The listing builds one solid part. Answer for the finished solid, in the listing's coordinates (mm). Coordinates: 2 decimals unless noted, no trailing zeros. Loops run counter-clockwise (first coordinate to the right, second up) from the corner with the lowest first, then second, coordinate; pieces in that order, holes last. Notation, with made-up numbers: M 31.5,-28 L 56.5,-28 A19 ccw 56.5,7 Z; hole C 42.25,13 d10. An arc over 180 degrees is marked long. Return JSON: item names as keys, results as strings. Group by question number.
1. Section A-A (y = -16) is taken. Write down the section's boundary in (x, z).
2. Section D-D (z = 4.1) is taken. Count the separate pieces of the cut face and the enclosed holes in it, then the cut area to 3 significant figures.
3. Given P1, Ø3.5, axis at x = 3.5, y = 1.5, coming from the +Z side, flat-ended and moving along its own axis, determine where the tip first touches the part or whether it passes through.
4. Straight lines are drawn through the part: L1, parallel to Y at x = 28, z = 3.2; L2, parallel to Y at x = 4, z = 2.1; L3, parallel to Y at x = -38.5, z = 4.05. For each, find the intervals that lie inside material, in ascending order. Write a range as from..to.
5. Section C-C (x = 15) is taken. Write down the section's boundary in (y, z).
6. Section B-B (x = -32) is taken. Write down the section's boundary in (y, z), then the cut area to 3 significant figures.
```python
from build123d import *

# Parameters (mm, degrees)
SKETCH_1_W          = 100
SKETCH_1_H          = 100
SKETCH_1_R          = 1.5
EXTRUDE_1_DEPTH     = 5
SKETCH_2_R          = 1
CUT_EXTRUDE_1_DEPTH = 71.887234394
SKETCH_3_R          = 3.5
CUT_EXTRUDE_2_DEPTH = 2
SKETCH_4_R          = 1.5
CUT_EXTRUDE_3_DEPTH = 10
SKETCH_5_R          = 1.5
CUT_EXTRUDE_4_DEPTH = 10
SKETCH_6_W          = 30
SKETCH_6_H          = 50
CUT_EXTRUDE_5_DEPTH = 10


with BuildPart() as part:
    # 草图1 → 凸台-拉伸1 (new body)
    with BuildSketch(Plane.XY):
        Rectangle(SKETCH_1_W, SKETCH_1_H)
        with Locations((-4, 0)):
            Circle(SKETCH_1_R, mode=Mode.SUBTRACT)
        with Locations(Location((4, 0, 0), (0, 0, 180))):
            Circle(SKETCH_1_R, mode=Mode.SUBTRACT)
    extrude(amount=EXTRUDE_1_DEPTH)

    # 草图2 → 切除-拉伸1 (cut, through all)
    with BuildSketch(Plane.XY.offset(5)):
        with Locations(Location((-46, -46, 0), (0, 0, 180))):
            Circle(SKETCH_2_R)
        with Locations((-46, 16)):
            Circle(SKETCH_2_R)
        with Locations((-4, -46)):
            Circle(SKETCH_2_R)
        with Locations((-4, 16)):
            Circle(SKETCH_2_R)
    extrude(amount=-CUT_EXTRUDE_1_DEPTH, mode=Mode.SUBTRACT)

    # 草图3 → 切除-拉伸2 (cut)
    with BuildSketch(Plane.XY.offset(5)):
        with Locations((-4, 0)):
            Circle(SKETCH_3_R)
        with Locations((4, 0)):
            Circle(SKETCH_3_R)
    extrude(amount=-CUT_EXTRUDE_2_DEPTH, mode=Mode.SUBTRACT)

    # 草图4 → 切除-拉伸3 (cut)
    with BuildSketch(Plane.XY.offset(5)):
        with Locations((35, 0)):
            Circle(SKETCH_4_R)
        with Locations((15, 0)):
            Circle(SKETCH_4_R)
        with Locations((35, -8)):
            Circle(SKETCH_4_R)
        with Locations((15, -8)):
            Circle(SKETCH_4_R)
        with Locations((35, -16)):
            Circle(SKETCH_4_R)
        with Locations((15, -16)):
            Circle(SKETCH_4_R)
        with Locations((35, -24)):
            Circle(SKETCH_4_R)
        with Locations((15, -24)):
            Circle(SKETCH_4_R)
        with Locations((35, -32)):
            Circle(SKETCH_4_R)
        with Locations((15, -32)):
            Circle(SKETCH_4_R)
        with Locations((35, -40)):
            Circle(SKETCH_4_R)
        with Locations((15, -40)):
            Circle(SKETCH_4_R)
    extrude(amount=-CUT_EXTRUDE_3_DEPTH, mode=Mode.SUBTRACT)

    # 草图5 → 切除-拉伸4 (cut)
    with BuildSketch(Plane(origin=(0, 0, 0), x_dir=(-1, 0, 0), z_dir=(0, 0, -1))):
        with Locations((35.821699256, 46)):
            Circle(SKETCH_5_R)
        with Locations((35.821699256, 26)):
            Circle(SKETCH_5_R)
        with Locations((27.821699256, 46)):
            Circle(SKETCH_5_R)
        with Locations((27.821699256, 26)):
            Circle(SKETCH_5_R)
        with Locations((19.821699256, 46)):
            Circle(SKETCH_5_R)
        with Locations((19.821699256, 26)):
            Circle(SKETCH_5_R)
        with Locations((11.821699256, 46)):
            Circle(SKETCH_5_R)
        with Locations((11.821699256, 26)):
            Circle(SKETCH_5_R)
        with Locations((3.821699256, 46)):
            Circle(SKETCH_5_R)
        with Locations((3.821699256, 26)):
            Circle(SKETCH_5_R)
        with Locations((-4.178300744, 46)):
            Circle(SKETCH_5_R)
        with Locations((-4.178300744, 26)):
            Circle(SKETCH_5_R)
        with Locations((-12.178300744, 46)):
            Circle(SKETCH_5_R)
        with Locations((-12.178300744, 26)):
            Circle(SKETCH_5_R)
        with Locations((-20.178300744, 46)):
            Circle(SKETCH_5_R)
        with Locations((-20.178300744, 26)):
            Circle(SKETCH_5_R)
        with Locations((-28.178300744, 46)):
            Circle(SKETCH_5_R)
        with Locations((-28.178300744, 26)):
            Circle(SKETCH_5_R)
        with Locations((-36.178300744, 46)):
            Circle(SKETCH_5_R)
        with Locations((-36.178300744, 26)):
            Circle(SKETCH_5_R)
        with Locations((-44.178300744, 46)):
            Circle(SKETCH_5_R)
        with Locations((-44.178300744, 26)):
            Circle(SKETCH_5_R)
    extrude(amount=-CUT_EXTRUDE_4_DEPTH, mode=Mode.SUBTRACT)

    # 草图6 → 切除-拉伸5 (cut)
    with BuildSketch(Plane(origin=(0, 0, 0), x_dir=(-1, 0, 0), z_dir=(0, 0, -1))):
        with Locations((25, -15)):
            Rectangle(SKETCH_6_W, SKETCH_6_H)
    extrude(amount=-CUT_EXTRUDE_5_DEPTH, mode=Mode.SUBTRACT)


solid = part.part
```
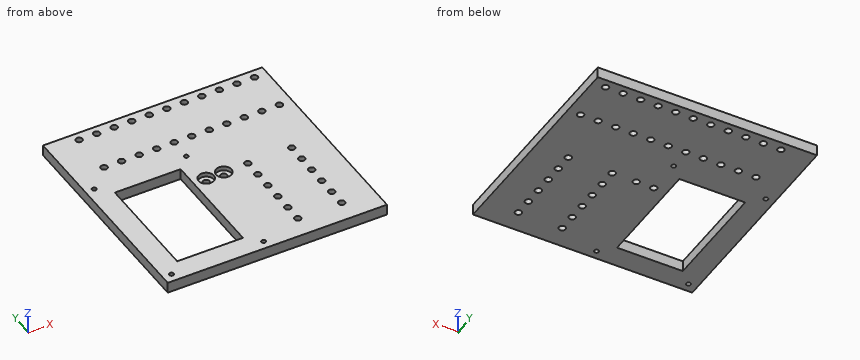
Worked out:
{
 "1": {"outline": "M -50,0 L -40,0 L -40,5 L -50,5 Z; M -10,0 L 13.5,0 L 13.5,5 L -10,5 Z; M 16.5,0 L 33.5,0 L 33.5,5 L 16.5,5 Z; M 36.5,0 L 50,0 L 50,5 L 36.5,5 Z"},
 "2": {"separate pieces": "1", "enclosed holes": "41", "area": "8,170 mm^2"},
 "3": {"P1": "z = 3"},
 "4": {"L1": "-50..24.51, 27.49..44.51, 47.49..50", "L2": "-50..-1.5, 1.5..24.51, 27.49..44.51, 47.49..50", "L3": "-50..-40, 10..50"},
 "5": {"outline": "M -50,0 L -41.5,0 L -41.5,5 L -50,5 Z; M -38.5,0 L -33.5,0 L -33.5,5 L -38.5,5 Z; M -30.5,0 L -25.5,0 L -25.5,5 L -30.5,5 Z; M -22.5,0 L -17.5,0 L -17.5,5 L -22.5,5 Z; M -14.5,0 L -9.5,0 L -9.5,5 L -14.5,5 Z; M -6.5,0 L -1.5,0 L -1.5,5 L -6.5,5 Z; M 1.5,0 L 50,0 L 50,5 L 1.5,5 Z"},
 "6": {"outline": "M -50,0 L -40,0 L -40,5 L -50,5 Z; M 10,0 L 50,0 L 50,5 L 10,5 Z", "area": "250 mm^2"}
}
